Verification items for the finished model (mm, model axes). Round coordinates to 2 decimals unless told otherwise and drop trailing zeros. Write each loop counter-clockwise with the first axis right and the second up, starting at its lowest first coordinate (ties: lowest second). Pieces come first, ordered by that corner, then holes. Notation, with made-up numbers: M -1.75,33.5 L 5.25,33.5 A26 ccw 5.25,72.5 Z; hole C -12,-28 d10. An arc over 180 degrees is marked long. One line per question, with ' | ' between items. Start each with the question number.
Q1. Cross-section at C-C (x = -75). Record the boundary of the cut face in (y, z).
Q2. Cross-section at D-D (y = 5.75). Record the boundary of the cut face in (x, z), then the cut area to 3 significant figures.
Q3. Cross-section at B-B (x = 0). Record the boundary of the cut face in (y, z), then the cut area to 3 significant figures.
Q4. Cross-section at A-A (z = 0). Record the boundary of the cut face in (x, y), then the cut area to 3 significant figures.
Q5. Gauge pin test, flat ends, axial feed: pin 1 (4 mm diameter, centred on x = 48, y = 8, fed in from +Z); pin 2 (18 mm diameter, centred on x = 0, z = 75, fed in from +Y); pin 3 (4 mm diameter, centred on y = 6.5, z = -51, fed in from +X); pin 4 (5 mm diameter, centred on y = 3.5, z = -37, fed in from +X). Record the tip position at first contact, or that the pin passes through.
Q6. Thickness scan on line 1 along X through (y, z) = (7, 0); line 2 along X through (y, z) = (2.5, 1); line 3 along Z through (x, y) = (-0.5, 4.5). Record the ranges inside material, lowest first. Write a range as from..to.
from build123d import *

# Parameters (mm, degrees)
SKETCH1_R           = 120
SKETCH1_R_2         = 10
BOSS_EXTRUDE1_DEPTH = 10


with BuildPart() as part:
    # Sketch1 → Boss-Extrude1 (new body)
    with BuildSketch(Plane(origin=(0, 0, 0), x_dir=(1, 0, 0), z_dir=(0, 1, 0))):
        with Locations(Location((0, 0, 0), (0, 0, 270))):
            Circle(SKETCH1_R)
        with Locations(Location((0, 0, 0), (0, 0, 270))):
            Circle(SKETCH1_R_2, mode=Mode.SUBTRACT)
        with Locations(Location((75, 0, 0), (0, 0, 270))):
            Circle(SKETCH1_R_2, mode=Mode.SUBTRACT)
        with Locations(Location((0, -75, 0), (0, 0, 270))):
            Circle(SKETCH1_R_2, mode=Mode.SUBTRACT)
        with Locations(Location((-75, 0, 0), (0, 0, 270))):
            Circle(SKETCH1_R_2, mode=Mode.SUBTRACT)
        with Locations(Location((0, 75, 0), (0, 0, 270))):
            Circle(SKETCH1_R_2, mode=Mode.SUBTRACT)
    extrude(amount=BOSS_EXTRUDE1_DEPTH)


solid = part.part
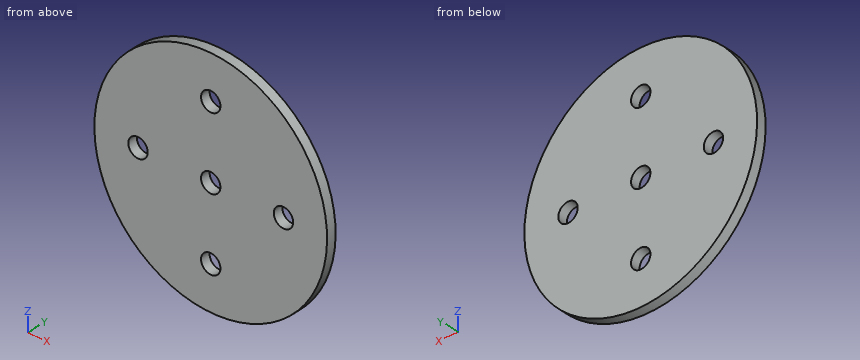
Determined:
1) outline: M 0,-93.67 L 10,-93.67 L 10,-10 L 0,-10 Z; M 0,10 L 10,10 L 10,93.67 L 0,93.67 Z
2) outline: C 0,0 d240; hole C -75,0 d20; hole C 0,-75 d20; hole C 0,0 d20; hole C 0,75 d20; hole C 75,0 d20 | area: 43,700 mm²
3) outline: M 0,-120 L 10,-120 L 10,-85 L 0,-85 Z; M 0,-65 L 10,-65 L 10,-10 L 0,-10 Z; M 0,10 L 10,10 L 10,65 L 0,65 Z; M 0,85 L 10,85 L 10,120 L 0,120 Z | area: 1,800 mm²
4) outline: M -120,0 L -85,0 L -85,10 L -120,10 Z; M -65,0 L -10,0 L -10,10 L -65,10 Z; M 10,0 L 65,0 L 65,10 L 10,10 Z; M 85,0 L 120,0 L 120,10 L 85,10 Z | area: 1,800 mm²
5) pin 1: stops at z = 110.83 | pin 2: passes through | pin 3: stops at x = 109.54 | pin 4: stops at x = 114.93
6) line 1: x = -120..-85, -65..-10, 10..65, 85..120 | line 2: x = -120..-84.95, -65.05..-9.95, 9.95..65.05, 84.95..120 | line 3: z = -120..-84.99, -65.01..-9.99, 9.99..65.01, 84.99..120
